The model under review builds one solid part; all positions refer to its coordinate system, in mm. Face numbers are marked on the shaded views. Coordinates: 2 decimals unless noted, no trailing zeros. Loops run counter-clockwise (first coordinate to the right, second up) from the corner with the lowest first, then second, coordinate; pieces in that order, holes last. Notation, with made-up numbers: M 74,53.5 L 96,53.5 A16 ccw 96,58.5 Z; hole C 37.25,65 d10. An arc over 180 degrees is marked long. Use CSV: the item, a comma, the result in double quotes. Start each with the question number.
1. Add section C-C, the plane z = 7.75. Write out the cut boundary in (x, y), then the cut area to 3 significant figures.
2. For L1, parallel to X at y = 0.75, z = 22; L2, parallel to Z at x = -29, y = 5; L3, parallel to X at y = 1.5, z = 9 (1 decimal), list the stretches that pass through material, from the lowest coordinate up.
3. Clearance check with flat-ended pins moving along their axes: P1, Ø6.5, axis at x = -6.37, z = 7.51, coming from the +Y side; P2, Ø12, axis at x = 37.5, z = 14.5, coming from the -Y side; P3, Ø2, axis at x = 68.5, z = 9.5, coming from the -Y side; P4, Ø1, axis at y = 4.5, z = 21.5, coming from the -X side. State where each tip first meets the part, or that it passes through.
4. Add section B-B, the plane y = 4.25. Write out the cut boundary in (x, z).
5. Draft analysis for pull direction Z (two halves, no side actions). For the marked faces 1 and 2, state which applies: +Z half, -Z half, draft (parallel to the pull), parting line (faces both ways), or undercut.
Autodesk Inventor part; units mm, degrees
ref_plane "YZ Plane" through (0, 0, 0) normal (1, 0, 0) x (0, 1, 0)
ref_plane "XZ Plane" through (0, 0, 0) normal (0, 1, 0) x (-1, 0, 0)
ref_plane "XY Plane" through (0, 0, 0) normal (0, 0, 1) x (1, 0, 0)
sketch "Sketch2" plane through (0, 0, 0) normal (0, 1, 0) x (-1, 0, 0)
  line L0 (0, 0) -> (60, 0)
  line L1 (60, 0) -> (60, 25)
  line L2 (60, 25) -> (0, 25)
  line L3 (0, 25) -> (0, 0)
  dimension "d2" = 25
  dimension "d3" = 60
extrude "Extrusion1" add sketch "Sketch2" along normal blind 3
sketch "Sketch4" plane through (0, 3, 0) normal (0, 1, 0) x (1, 0, 0)
  line L0 (-60, 0) -> (-60, -25) construction
  line L1 (-60, -12.5) -> (-56, -12.5) construction
  circle A0 centre (-54.0543, -17.5142) radius 2
  circle A1 centre (-54.0543, -7.5142) radius 2
  line L2 (-60, -25) -> (0, -25)
  line L3 (0, 0) -> (-60, 0)
  circle A2 centre (-6.3738, -17.5142) radius 2
  circle A3 centre (-6.3738, -7.5142) radius 2
  line L4 (-50, -21) -> (-9.77, -21)
  line L5 (-9.77, -21) -> (-9.77, -4)
  line L6 (-9.77, -4) -> (-50, -4)
  line L7 (-50, -4) -> (-50, -21)
  line L8 (-54.0543, -17.5142) -> (-51.0543, -17.5142)
  line L9 (-54.0543, -7.5142) -> (-51.0543, -7.5142)
  line L10 (-6.3738, -17.5142) -> (-9.3738, -17.5142)
  line L11 (-6.3738, -7.5142) -> (-9.3738, -7.5142)
  dimension "d8" = 4
  dimension "d9" = 4
  dimension "d11" = 40.23
  dimension "d12" = 3
  dimension "d13" = 3
  dimension "d14" = 3
  dimension "d15" = 3
hole "Hole1" at (-54.0543, 3, 17.5142) at (-54.0543, 3, 7.5142) at (-6.3738, 3, 17.5142) at (-6.3738, 3, 7.5142) direction (0, -1, 0) diameter 4 depth 8 tip angle 118
sketch "Sketch8" plane through (0, 3, 0) normal (0, 1, 0) x (1, 0, 0)
  circle A0 centre (-54.0543, -17.5142) radius 2
  line L0 (-54.0543, -17.5142) -> (-51.0543, -17.5142)
  circle A1 centre (-54.0543, -7.5142) radius 2
  line L1 (-54.0543, -7.5142) -> (-51.0543, -7.5142)
  circle A2 centre (-6.3738, -17.5142) radius 2
  line L2 (-6.3738, -17.5142) -> (-9.3738, -17.5142)
  circle A3 centre (-6.3738, -7.5142) radius 2
  line L3 (-6.3738, -7.5142) -> (-9.3738, -7.5142)
  line L4 (-51.1048, -22.3867) -> (-10.1048, -22.3867)
  line L5 (-10.1048, -22.3867) -> (-10.1048, -2.3867)
  line L6 (-10.1048, -2.3867) -> (-51.1048, -2.3867)
  line L7 (-51.1048, -2.3867) -> (-51.1048, -22.3867)
  point P0 (0, 0)
  dimension "d23" = 3
  dimension "d24" = 3
  dimension "d25" = 3
  dimension "d26" = 3
  dimension "d27" = 20
  dimension "d30" = 41
extrude "Extrusion2" cut sketch "Sketch8" against normal blind 3 contours L7 L6 L5 L4
sketch "Sketch10" plane through (0, 3, 0) normal (0, 1, 0) x (1, 0, 0)
  line L0 (0, -25) -> (0, 0)
  line L1 (-60, -25) -> (0, -25)
  line L2 (0, -25) -> (0, -22.3867)
  line L3 (0, -22.3867) -> (-60, -22.3867)
  line L4 (-60, -22.3867) -> (-60, -25)
  line L5 (-60, 0) -> (0, 0)
  line L6 (0, 0) -> (0, -2.3796)
  line L7 (0, -2.3796) -> (-60, -2.3796)
  line L8 (-60, -2.3796) -> (-60, 0)
extrude "Extrusion3" add sketch "Sketch10" along normal blind 4 and the other way blind 3
sketch "Sketch11" plane through (0, 0, 0) normal (0, -1, 0) x (1, 0, 0)
  line L0 (0, 0) -> (66, 0)
  line L1 (0, 25) -> (66, 25)
  line L2 (66, 0) -> (66, 25)
  line L3 (0, 0) -> (0, 25)
  line L4 (0, 25) -> (0, 0)
  dimension "d39" = 66
extrude "Extrusion4" add sketch "Sketch11" against normal blind 7
sketch "Sketch12" plane through (66, 0, 25) normal (1, 0, 0) x (0, 0, -1)
  line L0 (0, 0) -> (0, 7) construction
  line L1 (0, 0) -> (0, 7) construction
  line L2 (0, 3.5) -> (25, 3.5) construction
  line L3 (25, 0) -> (25, 7) construction
  line L4 (2.6133, 0) -> (22.6133, 0) construction
  line L5 (12.6133, 0) -> (12.6169, 7) construction
  line L6 (22.6204, 7) -> (2.6133, 7) construction
  line L7 (2.8651, 0.55) -> (22.3651, 0.55)
  line L8 (22.3651, 0.55) -> (22.3651, 6.45)
  line L9 (22.3651, 6.45) -> (2.8651, 6.45)
  line L10 (2.8651, 6.45) -> (2.8651, 0.55)
  line L11 (12.6151, 0.55) -> (12.6151, 6.45) construction
  line L12 (2.8651, 3.5) -> (22.3651, 3.5) construction
  point P0 (12.6151, 3.5)
  dimension "d42" = 19.5
  dimension "d43" = 5.9
extrude "Extrusion5" add sketch "Sketch12" along normal blind 4
properties part number "servo_holder"
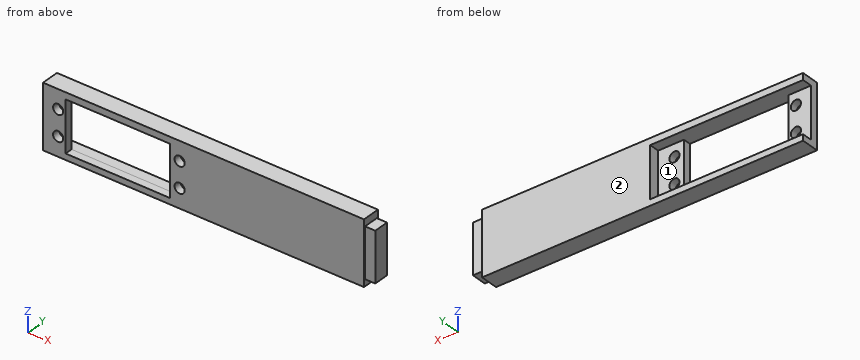
Computed:
1,outline,"M -60,0 L -56.04,0 L -56.04,3 L -60,3 Z; M -52.07,0 L -51.1,0 L -51.1,3 L -52.07,3 Z; M -10.1,0 L -8.36,0 L -8.36,3 L -10.1,3 Z; M -4.39,0 L 66,0 L 66,0.55 L 70,0.55 L 70,6.45 L 66,6.45 L 66,7 L 0,7 L 0,3 L -4.39,3 Z"
1,area,"519 mm^2"
2,L1,"x = -60 to -51.1, -10.1 to 70"
2,L2,"z = 0 to 2.38, 22.39 to 25"
2,L3,"x = -60 to -55.4, -52.7 to -51.1, -10.1 to -7.7, -5 to 70"
3,P1,"stops at y = 3"
3,P2,"stops at y = 0"
3,P3,"stops at y = 0.55"
3,P4,"stops at x = 0"
4,outline,"M -60,0 L 66,0 L 66,2.63 L 70,2.63 L 70,22.13 L 66,22.13 L 66,25 L -60,25 L -60,22.39 L 0,22.39 L 0,2.38 L -60,2.38 Z"
5,face 1,"undercut"
5,face 2,"draft"
